Can you work these out from the model? Positions are in its coordinate system, mm. Face numbers are marked on the shaded views. Give positions to 0.01 mm unless a question says otherwise; leave off trailing zeros. Loops run counter-clockwise (first coordinate to the right, second up) from the corner with the lowest first, then second, coordinate; pieces in that order, holes last. Notation, with made-up numbers: (76, 77) - (116, 77) arc R17 ccw to (116, 104) - close; hole circle Ø9 at (77.25, 54). An arc over 180 degrees is marked (long way). Answer as a JSON object with one key per item and string values.
```python
from build123d import *

# Parameters (mm, degrees)
F1_DEPTH = 600
F4_DEPTH = 6
F6_DEPTH = 6
F7_R     = 6.5
F8_DEPTH = 25
F3_R     = 10
F9_DEPTH = 25


with BuildPart() as f1:
    # F0 (on Front) → F1 (new body)
    with BuildSketch(Plane.XZ):
        Polygon((3.163387, -4.385628), (3.163387, -10.385628), (66.627489, -10.385628), (98.35954, 44.575896), (93.163387, 47.575896), (63.163387, -4.385628), align=None)
    extrude(amount=F1_DEPTH)

    # F2 (on face) → F4 (join)
    with BuildSketch(Plane(origin=(0, 0, 0), x_dir=(-1, 0, 0), z_dir=(0, 1, 0))):
        Polygon((-3.163387, -10.385628), (-3.163387, 1.614372), (-87.967235, 50.575896), (-98.35954, 44.575896), (-66.627489, -10.385628), align=None)
    extrude(amount=F4_DEPTH)

    # F5 (on face) → F6 (join)
    with BuildSketch(Plane.XZ.offset(600)):
        Polygon((3.163387, 11.614372), (3.163387, -10.385628), (66.627489, -10.385628), (98.35954, 44.575896), (79.351506, 55.652657), align=None)
    extrude(amount=F6_DEPTH)

    # F7 (on face) → F8 (cut)
    with BuildSketch(Plane.XZ.offset(606)):
        with Locations((70.307284, 31.987963)):
            Circle(F7_R)
        with Locations((28.163387, 7.614372)):
            Circle(F7_R)
    extrude(amount=-F8_DEPTH, mode=Mode.SUBTRACT)

    # F3 (on face) → F9 (cut)
    with BuildSketch(Plane.XY.offset(-4.385628)):
        with Locations((33.163387, -40)):
            Circle(F3_R)
        with Locations((33.163387, -120)):
            Circle(F3_R)
        with Locations((33.163387, -200)):
            Circle(F3_R)
        with Locations((33.163387, -280)):
            Circle(F3_R)
        with Locations((33.163387, -360)):
            Circle(F3_R)
        with Locations((33.163387, -440)):
            Circle(F3_R)
        with Locations((33.163387, -520)):
            Circle(F3_R)
    extrude(amount=-F9_DEPTH, mode=Mode.SUBTRACT)


solid = f1.part
```
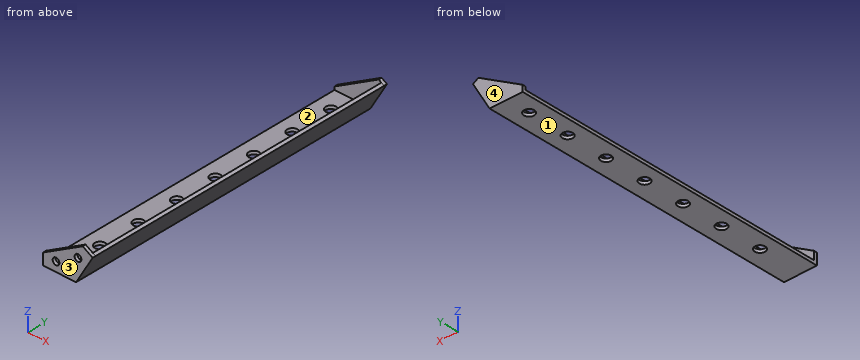
1) I'm going to push flat-ended pins straight in: P1, Ø23, axis at x = 33.16, y = -360, coming from the -Z side; P2, Ø8, axis at y = -316.5, z = 44, coming from the -X side; P3, Ø1, axis at y = -392, z = 41.5, coming from the -X side; P4, Ø10, axis at x = 61.5, y = -417, coming from the +Z side. Where does each tip first touch, or does it pass through?
Check sheet entries:
{"P1": "z = -10.39", "P2": "x = 88.79", "P3": "x = 89.37", "P4": "z = 1.39"}
2) Imagine slicing it at B-B on y = -494. Write out the boundary of the cut face in (x, z).
Check sheet entries:
{"outline": "(3.16, -10.39) - (66.63, -10.39) - (98.36, 44.58) - (93.16, 47.58) - (63.16, -4.39) - (3.16, -4.39) - close"}
3) I need wall thicknesses on L1, parallel to Y at x = 47.5, z = -2.5; L2, parallel to Y at x = 77, z = 45.5; L3, parallel to Z at x = 14, y = -466.5. Which ranges of each line are inside material? Lowest first, please.
Check sheet entries:
{"L1": "-606 to -600, 0 to 6", "L2": "-606 to -600", "L3": "-10.39 to -4.39"}
4) Imagine slicing it at A-A on y = -200. Write out the boundary of the cut face in (x, z).
Check sheet entries:
{"outline": "(3.16, -10.39) - (23.16, -10.39) - (23.16, -4.39) - (3.16, -4.39) - close; (43.16, -10.39) - (66.63, -10.39) - (98.36, 44.58) - (93.16, 47.58) - (63.16, -4.39) - (43.16, -4.39) - close"}
5) If we mould it in two halves opening along Y, with no side actions, what happens to the marked faces 1, 2, 3 and 4? For each: released by +Y, released by -Y, zero draft, split by the parting line, or undercut.
Check sheet entries:
{"face 1": "zero draft", "face 2": "undercut", "face 3": "released by -Y", "face 4": "released by +Y"}
